Model file for the job. Use its own axes, mm. A direction names the side the tool comes from. Give positions to 0.01 mm unless a question says otherwise; leave off trailing zeros. Write each loop counter-clockwise with the first axis right and the second up, starting at its lowest first coordinate (ties: lowest second). Pieces come first, ordered by that corner, then holes. Notation, with made-up numbers: (-4.5, -6) - (18.5, -6) arc R26 ccw to (18.5, 31) - close; hole circle Ø2 at (45, 75). An arc over 180 degrees is marked (long way). One line per item, written item: value. Start each with the question number.
(1) 3-axis set-ups, long thin cutter, end or side, ignore diameter. For faces 4 (the face through (50.8, -6.88, 34)), 5 (the face through (38.28, -13.53, 37.39)), 6 (the face through (25.4, -18, 26)): which of +Z, -Z, +X, -X, +Y, -Y reach the whole face in a straight line?
(2) Cut at C-C, the plane y = -20.25. List the corners of the cut face in (x, z).
(3) Cut at A-A, the plane x = 61. List the corners of the cut face in (y, z).
(4) Drop flat-ended pins along their axis: P1, Ø7.5, axis at y = -7, z = 29.5, coming from the +X side; P2, Ø11.5, axis at x = 63.5, y = -12.7, coming from the -Z side (3 decimals); P3, Ø2, axis at y = -12.5, z = 23.5, coming from the -X side; P4, Ø8, axis at x = 63, y = -18, coming from the +Z side. Give the stop position or say it passes through.
(5) Cut at D-D, the plane x = 27.5. List the corners of the cut face in (y, z), and give its area (3 significant figures).
(6) Mould opens along X. For faces 1 (the face through (0.02, -12.98, 9.66)), 2 (the face through (38, -25.4, 12)), 3 (the face through (11.34, -18.9, 9.66)) say: pulls with the +X half, pulls with the -X half, needs draft (parallel to the pull), parting line crosses it, or undercut.
(7) Cut at B-B, the plane z = 36. List the corners of the cut face in (x, y), and give its area (3 significant figures).
(8) Probe L1, parallel to Y at x = 63.5, z = 11; L2, parallel to Z at x = 35.75, y = -12.7; L3, parallel to Z at x = 13, y = -22.5. List the from-to ranges inside material, lowest first.
from build123d import *

# Parameters (mm, degrees)
F1_DEPTH = 25.4
F2_R     = 6.35
F3_DEPTH = 25.4
F4_R     = 6.35
F5_DEPTH = 25.4
F7_DEPTH = 25.4


with BuildPart() as f1:
    # F0 (on Front) → F1 (new body)
    with BuildSketch(Plane.XZ):
        Polygon((0, 19.05), (0, 0), (76.2, 0), (76.2, 19.05), (50.8, 19.05), (50.8, 43.9752354272), (25.4, 43.9752354272), (25.4, 19.05), align=None)
    extrude(amount=F1_DEPTH)

    # F2 (on face) → F3 (cut)
    with BuildSketch(Plane.YZ.offset(50.8)):
        with Locations((-12.7, 31.0931869331)):
            Circle(F2_R)
        with BuildLine():
            ThreePointArc((-25.4, 31.5126177136), (-12.7, 43.8001111156), (0, 31.5126177136))
            Line((0, 31.5126177136), (0, 43.9752354272))
            Line((0, 43.9752354272), (-25.4, 43.9752354272))
            Line((-25.4, 43.9752354272), (-25.4, 31.5126177136))
        make_face()
    extrude(amount=-F3_DEPTH, mode=Mode.SUBTRACT)

    # F4 (on face) → F5 (cut)
    with BuildSketch(Plane.XY.offset(19.05)):
        with Locations((12.7164462461, -12.7)):
            Circle(F4_R)
        with BuildLine():
            ThreePointArc((12.7, -25.4), (0.0164355973, -12.7), (12.7, 0))
            Line((12.7, 0), (0, 0))
            Line((0, 0), (0, -25.4))
            Line((0, -25.4), (12.7, -25.4))
        make_face()
        with Locations((63.5, -12.7)):
            Circle(F4_R)
    extrude(amount=-F5_DEPTH, mode=Mode.SUBTRACT)

    # F6 (on face) → F7 (cut)
    with BuildSketch(Plane.XY.offset(19.05)):
        with BuildLine():
            ThreePointArc((63.5, 0), (72.4802561211, -3.7197438789), (76.2, -12.7))
            Line((76.2, -12.7), (76.2, 0))
            Line((76.2, 0), (63.5, 0))
        make_face()
        with BuildLine():
            ThreePointArc((76.2, -12.7), (72.4802561211, -21.6802561211), (63.5, -25.4))
            Line((63.5, -25.4), (76.2, -25.4))
            Line((76.2, -25.4), (76.2, -12.7))
        make_face()
    extrude(amount=-F7_DEPTH, mode=Mode.SUBTRACT)


solid = f1.part
Answers follow:
1. face 4: +Z, +X, +Y, -Y
1. face 5: +X, -X
1. face 6: +Z, -X, +Y, -Y
2. outline: (2.5, 0) - (73.71, 0) - (73.71, 19.05) - (50.8, 19.05) - (50.8, 41.31) - (25.4, 41.31) - (25.4, 19.05) - (2.5, 19.05) - close
3. outline: (-25.4, 0) - (-18.54, 0) - (-18.54, 19.05) - (-25.4, 19.05) - close; (-6.86, 0) - (0, 0) - (0, 19.05) - (-6.86, 19.05) - close
4. P1: stops at x = 50.8
4. P2: passes through
4. P3: stops at x = 25.4
4. P4: stops at z = 19.05
5. outline: (-25.4, 0) - (0, 0) - (0, 31.51) arc R12.71 ccw to (-25.4, 31.51) - close; hole circle Ø12.7 at (-12.7, 31.09)
5. area: 917 mm²
6. face 1: pulls with the -X half
6. face 2: needs draft
6. face 3: undercut
7. outline: (25.4, -24.42) - (50.8, -24.42) - (50.8, -16.73) - (25.4, -16.73) - close; (25.4, -8.67) - (50.8, -8.67) - (50.8, -0.98) - (25.4, -0.98) - close
7. area: 391 mm²
8. L1: y = -25.4 to -19.05, -6.35 to 0
8. L2: z = 0 to 24.74, 37.44 to 43.8
8. L3: z = 0 to 19.05
